Work out the finished part from the listing and answer in its coordinate system (mm). Round coordinates to 2 decimals unless told otherwise and drop trailing zeros. Write each loop counter-clockwise with the first axis right and the second up, starting at its lowest first coordinate (ties: lowest second). Pieces come first, ordered by that corner, then holes.
1. Find section C-C (y = 0.5). Count the separate pieces of the cut face and the enclosed holes in it, and give its area (3 significant figures).
2. Find section B-B (x = 0). Write down the section's boundary in (y, z), and give its area (3 significant figures).
3. Find section A-A (z = 34.6). Write down the section's boundary in (x, y) (3 decimals).
4. A flat-ended cylindrical pin translates along its axis: pin 1 Ø1.9 at (x, z) = (-7.525, 34.6) entering from -Y. Find the tip coordinate at first contact, or state that the pin passes through.
5. Find section D-D (z = -32). Write down the section's boundary in (x, y).
6. Straight lines are drawn through the part: probe 1 along X at (y, z) = (1, -25); probe 2 along X at (y, z) = (0.45, 19.5) (3 decimals); probe 3 along Z at (x, y) = (-7.25, 0.2). For each, find the intervals that lie inside material, in ascending order.
Autodesk Inventor part; units mm, degrees
ref_plane "YZ Plane" through (0, 0, 0) normal (1, 0, 0) x (0, 1, 0)
ref_plane "XZ Plane" through (0, 0, 0) normal (0, 1, 0) x (-1, 0, 0)
ref_plane "XY Plane" through (0, 0, 0) normal (0, 0, 1) x (1, 0, 0)
sketch "Sketch1" plane through (0, 0, 0) normal (0, 1, 0) x (-1, 0, 0)
  line L0 (10, -35) -> (-10, -35)
  line L1 (-10, -35) -> (-10, 41.4211)
  line L2 (10, 41.4211) -> (10, -35)
  arc A0 (-10, 41.4211) -> (10, 41.4211) centre (0, 47.1) ccw
  point P0 (0, 0)
  dimension "d2" = 35
  dimension "d3" = 10
  dimension "d36" = 23
  dimension "d37" = 82.1
  dimension "d39" = 76.4211
  dimension "d40" = 20
extrude "Plate1" add sketch "Sketch1" along normal blind 1.5
sketch "Sketch3" plane through (0, 1.5, 0) normal (0, 1, 0) x (1, 0, 0)
  circle A0 centre (0, 25) radius 10
  circle A1 centre (0, -25) radius 10
  line L0 (-10, 35) -> (10, 35)
  line L1 (10, -44) -> (-10, -44)
  line L2 (-10, 35) -> (10, 35)
  line L3 (10, 35) -> (10, 25)
  line L4 (10, 25) -> (-10, 25)
  line L5 (-10, 25) -> (-10, 35)
  line L6 (10, -35) -> (-10, -35)
  line L7 (-10, -35) -> (-10, -25)
  line L8 (-10, -25) -> (10, -25)
  line L9 (10, -25) -> (10, -44)
  point P0 (0, 0)
  point P1 (-10, -41.4211)
  point P2 (10, -25)
  point P3 (0, -35)
  point P4 (-10, -35)
  point P5 (0, 35)
  point P6 (10, 35)
  dimension "d12" = 20
  dimension "d13" = 20
  dimension "d14" = 10
  dimension "d15" = 10
  dimension "d16" = 25
  dimension "d17" = 25
  dimension "d18" = 10
extrude "Extrusion1" cut sketch "Sketch3" against normal blind 10 contours L5 L0 A0 | A0 L0 L3
sketch "Sketch4" plane through (0, 1.5, 0) normal (0, 1, 0) x (1, 0, 0)
  circle A0 centre (-7, 25) radius 0.8
  arc A1 (10, 25) -> (-10, 25) centre (0, 25) ccw
  circle A2 centre (0, 18) radius 0.8
  circle A3 centre (7, 25) radius 0.8
  circle A4 centre (0, 32) radius 0.8
  point P0 (0, 0)
  dimension "d21" = 0
  dimension "d22" = 7
  dimension "d23" = 1.6
  dimension "d26" = 360
hole "Hole2" at (0, 1.5, -32) at (7, 1.5, -25) at (0, 1.5, -18) at (-7, 1.5, -25) direction (0, -1, 0) diameter 2.1 depth 1.5
fillet "Fillet1" radius 1 2 edges at (-10, 0.75, 41.4211) (10, 0.75, 41.4211)
sketch "Sketch5" plane through (0, 1.5, 0) normal (0, 1, 0) x (1, 0, 0)
  arc A0 (10, 25) -> (-10, 25) centre (0, 25) ccw
  point P0 (0, 0)
hole "Hole3" at (0, 1.5, -25) direction (0, -1, 0) diameter 7.2 depth 1.5
sketch "Sketch8" plane through (0, 1.5, 0) normal (0, 1, 0) x (1, 0, 0)
  line L0 (19.8447, -22.3636) -> (-14.9774, -42.4682)
  arc A0 (8.28, -39.1193) -> (-8.28, -39.1193) centre (0, -47.1) ccw
  arc A1 (8.28, -39.1193) -> (10, -38.4253) centre (9, -38.4253) ccw
  line L1 (10, 25) -> (10, -38.4253)
  point P0 (0, 0)
  point P1 (10, -28.0474)
  point P2 (-5.75, -37.1407)
  dimension "d63" = 60
extrude "Extrusion2" cut sketch "Sketch8" against normal blind 1.5
sketch "Sketch9" plane through (0, 0, 0) normal (0, -1, 0) x (1, 0, 0)
  circle A0 centre (-7.525, 34.6) radius 1.05
  circle A1 centre (7.525, 19.5) radius 1.05
  circle A2 centre (7.525, 19.5) radius 1.05
  line L0 (-10, -25) -> (-10, 38.4253)
  circle A3 centre (-7.525, 19.5) radius 1.05
  point P0 (0, 0)
hole "Hole6" at (-7.525, 0, 19.5) at (7.525, 0, 19.5) at (-7.525, 0, 34.6) direction (0, 1, 0) diameter 2.1 end through all
equation "\"d33\" = Thickness"
equation "\"d47\" = Thickness"
equation "\"d71\" = Thickness"
equation "\"d4\" = Thickness"
equation "\"BendReliefWidth\" = Thickness"
equation "\"BendReliefDepth\" = 0.5 * Thickness"
equation "\"CornerReliefSize\" = 4 * Thickness"
equation "\"MinimumRemnant\" = 2 * Thickness"
equation "\"TransitionRadius\" = BendRadius"
equation "\"JacobiRadiusSize\" = BendRadius"
equation "\"GapSize\" = Thickness"
properties part number "axis_8_10_connector_frame" material "Aluminum 6061-AHC"
Worked answers:
1. separate pieces: 1
1. enclosed holes: 8
1. area: 1,270 mm2
2. outline: (0, -35) - (1.5, -35) - (1.5, -33.05) - (0, -33.05) - close; (0, -30.95) - (1.5, -30.95) - (1.5, -28.6) - (0, -28.6) - close; (0, -21.4) - (1.5, -21.4) - (1.5, -19.05) - (0, -19.05) - close; (0, -16.95) - (1.5, -16.95) - (1.5, 33.82) - (0, 33.82) - close
2. area: 86.1 mm2
3. outline: (-10, 0) - (-8.575, 0) - (-8.575, 1.5) - (-10, 1.5) - close; (-6.475, 0) - (-1.349, 0) - (-1.349, 1.5) - (-6.475, 1.5) - close
4. pin 1: passes through
5. outline: (-7.14, 0) - (-1.05, 0) - (-1.05, 1.5) - (-7.14, 1.5) - close; (1.05, 0) - (7.14, 0) - (7.14, 1.5) - (1.05, 1.5) - close
6. probe 1: x = -10 to -8.05, -5.95 to -3.6, 3.6 to 5.95, 8.05 to 10
6. probe 2: x = -10 to -8.575, -6.475 to 6.475, 8.575 to 10
6. probe 3: z = -31.89 to -26.02, -23.98 to 18.49, 20.51 to 33.59, 35.61 to 38.17
